Geometry check sheet. Reference: the model listing, model coordinates, mm. Coordinates: 2 decimals unless noted, no trailing zeros. Write each loop counter-clockwise with the first axis right and the second up, starting at its lowest first coordinate (ties: lowest second). Pieces come first, ordered by that corner, then holes. Notation, with made-up numbers: M 76.25,10 L 111.25,10 A25 cw 111.25,22 Z; hole C 34,-5.5 d9. An arc over 180 degrees is marked long. Answer as a JSON object with one key per item and string values. Group by question number.
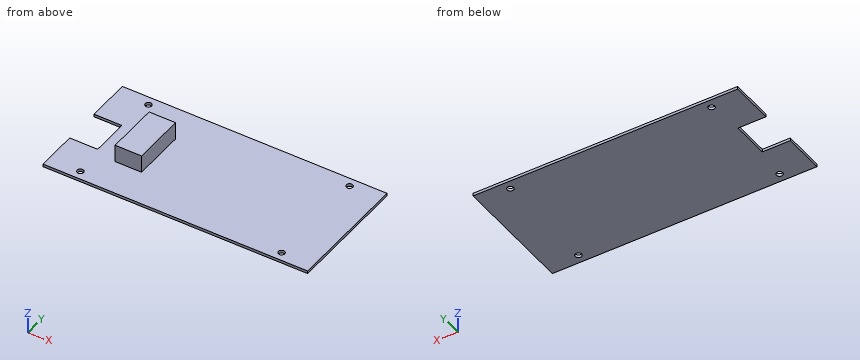
```python
from build123d import *

# Parameters (mm, degrees)
SKETCH_1_W          = 150
SKETCH_1_H          = 70
EXTRUDE_1_DEPTH     = 1.6
HOLE_WIZARD_M3_1_D  = 3.6
SKETCH_5_W          = 35.774901566
SKETCH_5_H          = 21.448543783
CUT_EXTRUDE_1_DEPTH = 10
SKETCH_6_W          = 15
SKETCH_6_H          = 30
EXTRUDE_2_DEPTH     = 10


with BuildPart() as part:
    # ｽｹｯﾁ1 → ﾎﾞｽ - 押し出し1 (new body)
    with BuildSketch(Plane.XY):
        Rectangle(SKETCH_1_W, SKETCH_1_H)
    extrude(amount=EXTRUDE_1_DEPTH)

    # M3 すきま穴1 (through all)
    with Locations(Plane.XY.offset(1.6)):
        with Locations((57, 30), (57, -30), (-57, -30), (-57, 30)):
            Hole(HOLE_WIZARD_M3_1_D / 2)

    # ｽｹｯﾁ5 → ｶｯﾄ - 押し出し1 (cut)
    with BuildSketch(Plane.XY.offset(1.6)):
        with Locations((-77.011061726, -0.754700365)):
            Rectangle(SKETCH_5_W, SKETCH_5_H)
    extrude(amount=-CUT_EXTRUDE_1_DEPTH, mode=Mode.SUBTRACT)

    # ｽｹｯﾁ6 → ﾎﾞｽ - 押し出し2 (add)
    with BuildSketch(Plane.XY.offset(1.6)):
        with Locations((-39.605094466, 0.185984115)):
            Rectangle(SKETCH_6_W, SKETCH_6_H)
    extrude(amount=EXTRUDE_2_DEPTH)


solid = part.part
```
1) Section check D-D (y = 25.5). Record the cut outline in (x, z), then the cut area to 3 significant figures.
2) Material ranges on probe 1 along Y at (x, z) = (-57, 1.15); probe 2 along X at (y, z) = (11, 4.75); probe 3 along Z at (x, y) = (-49.5, 5), recorded low to high. Write a range as [from, to].
3) Go/stop test with flat-tipped pins: pin 1 Ø6 at (x, z) = (-33.5, 2.5) entering from -Y; pin 2 Ø3 at (x, y) = (-57, -30) entering from -Z; pin 3 Ø0.5 at (y, z) = (-3.5, 0.5) entering from -X; pin 4 Ø3 at (x, z) = (-36, 8) entering from -Y. Record where each tip stops, or that it passes through.
4) Section check A-A (y = -30). Record the cut outline in (x, z).
5) Section check B-B (x = 57). Record the cut outline in (y, z).
6) Section check C-C (z = 5.25). Record the cut outline in (x, y).
Entries:
{
 "1": {"outline": "M -75,0 L 75,0 L 75,1.6 L -75,1.6 Z", "area": "240 mm^2"},
 "2": {"probe 1": "[-35, -31.8], [-28.2, 28.2], [31.8, 35]", "probe 2": "[-47.11, -32.11]", "probe 3": "[0, 1.6]"},
 "3": {"pin 1": "y = -35", "pin 2": "through", "pin 3": "x = -59.12", "pin 4": "y = -14.81"},
 "4": {"outline": "M -75,0 L -58.8,0 L -58.8,1.6 L -75,1.6 Z; M -55.2,0 L 55.2,0 L 55.2,1.6 L -55.2,1.6 Z; M 58.8,0 L 75,0 L 75,1.6 L 58.8,1.6 Z"},
 "5": {"outline": "M -35,0 L -31.8,0 L -31.8,1.6 L -35,1.6 Z; M -28.2,0 L 28.2,0 L 28.2,1.6 L -28.2,1.6 Z; M 31.8,0 L 35,0 L 35,1.6 L 31.8,1.6 Z"},
 "6": {"outline": "M -47.11,-14.81 L -32.11,-14.81 L -32.11,15.19 L -47.11,15.19 Z"}
}
